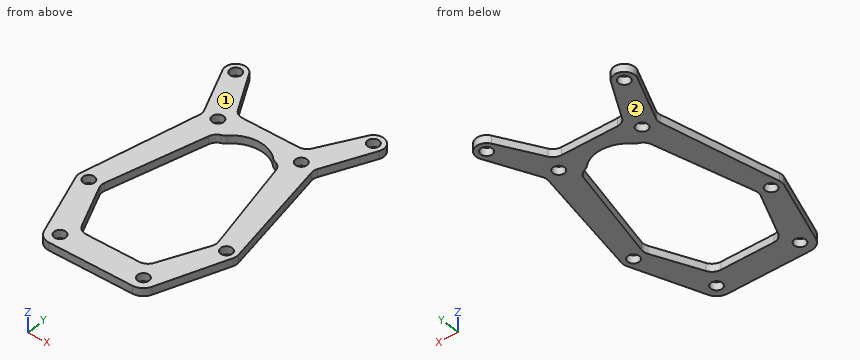
Autodesk Inventor part; units mm, degrees
ref_plane "YZ Plane" through (0, 0, 0) normal (1, 0, 0) x (0, 1, 0)
ref_plane "XZ Plane" through (0, 0, 0) normal (0, 1, 0) x (-1, 0, 0)
ref_plane "XY Plane" through (0, 0, 0) normal (0, 0, 1) x (1, 0, 0)
sketch "スケッチ1" plane through (0, 0, 0) normal (0, 0, 1) x (1, 0, 0)
  circle A0 centre (4, -6) radius 1.05
  circle A1 centre (4, -6) radius 1.1
  circle A2 centre (20, -6) radius 1.05
  circle A3 centre (20, -42) radius 1.1
  circle A4 centre (4, -42) radius 1.05
  circle A5 centre (20, -6) radius 1.1
  circle A6 centre (20, -42) radius 1.1
  circle A7 centre (4, -42) radius 1.1
  circle A8 centre (4, -42) radius 2.5
  circle A9 centre (20, -42) radius 2.5
  circle A10 centre (20, -6) radius 2.5
  circle A11 centre (4, -6) radius 2.5
  arc A12 (-0.741742, -29.885509) -> (-0.741742, -28.614491) centre (-1.2, -29.25) ccw
  arc A13 (24.741742, -28.614491) -> (24.741742, -29.885509) centre (25.2, -29.25) ccw
  arc A14 (-0.741742, 3.614491) -> (-0.741742, 4.885509) centre (-1.2, 4.25) ccw
  arc A15 (24.741742, 4.885509) -> (24.741742, 3.614491) centre (25.2, 4.25) ccw
  line L0 (24.741742, 5.75) -> (24.741742, 4.885509)
  line L1 (24.741742, 5.75) -> (22.7, 5.75)
  line L2 (22.7, 5.75) -> (22.7, 2.75)
  line L3 (24.741742, 2.75) -> (22.7, 2.75)
  line L4 (24.741742, 3.614491) -> (24.741742, 2.75)
  circle A16 centre (-1.2, 4.25) radius 1.1
  circle A17 centre (25.2, 4.25) radius 1.1
  circle A18 centre (25.2, -29.25) radius 1.1
  circle A19 centre (-1.2, -29.25) radius 1.1
  circle A20 centre (-1.2, -29.25) radius 2
  circle A21 centre (25.2, -29.25) radius 2
  circle A22 centre (25.2, 4.25) radius 2
  circle A23 centre (-1.2, 4.25) radius 2
  line L5 (-3.078107, -29.937542) -> (1.652366, -42.859427)
  line L6 (0.623256, -28.427966) -> (6.279069, -40.972458)
  line L7 (4, -39.5) -> (20, -39.5)
  line L8 (20, -44.5) -> (4, -44.5)
  line L9 (0.742189, -29.727393) -> (6.427736, -6.596741)
  line L10 (-3.160511, -28.854531) -> (1.549361, -5.505664)
  line L11 (-3.021278, 3.423595) -> (1.723402, -7.033006)
  line L12 (6.17819, -4.773016) -> (0.542552, 5.231587)
  line L13 (4, -3.5) -> (20, -3.5)
  line L14 (20, -8.5) -> (4, -8.5)
  line L15 (17.82181, -4.773016) -> (23.457448, 5.231587)
  line L16 (27.021278, 3.423595) -> (22.276598, -7.033006)
  line L17 (17.572264, -6.596741) -> (23.257811, -29.727393)
  line L18 (27.160511, -28.854531) -> (22.450639, -5.505664)
  line L19 (23.376744, -28.427966) -> (17.720931, -40.972458)
  line L20 (27.078107, -29.937542) -> (22.347634, -42.859427)
  circle A24 centre (12, -12.5) radius 6.232545
  point P0 (0, 0)
  point P1 (5.615196, -39.5)
  point P2 (0.906933, -29.057158)
  point P3 (5.959912, -8.5)
  point P4 (18.040088, -8.5)
  point P5 (23.093067, -29.057158)
  point P6 (18.384804, -39.5)
  point P7 (18.538906, -3.5)
  point P8 (5.461094, -3.5)
  point P9 (1.389644, -6.29745)
  point P10 (22.610356, -6.29745)
  point P11 (7.220396, -8.5)
  point P12 (16.779604, -8.5)
  dimension "d0" = 2.2
  dimension "d1" = 2.2
  dimension "d2" = 2.2
  dimension "d3" = 2.2
  dimension "d4" = 5
  dimension "d5" = 5
  dimension "d6" = 5
  dimension "d7" = 5
  dimension "d8" = 2.2
  dimension "d9" = 2.2
  dimension "d10" = 2.2
  dimension "d11" = 2.2
  dimension "d12" = 4
  dimension "d13" = 4
  dimension "d14" = 4
  dimension "d15" = 4
sketch "スケッチ1 outline for 押し出し1" plane through (0, 0, 0) normal (0, 0, 1) x (1, 0, 0)
  arc A0 (27.021278, 3.423595) -> (23.457448, 5.231587) centre (25.2, 4.25) ccw
  line L0 (22.610356, -6.29745) -> (27.021278, 3.423595)
  line L1 (23.457448, 5.231587) -> (18.538906, -3.5)
  line L2 (27.160511, -28.854531) -> (22.610356, -6.29745)
  line L3 (18.538906, -3.5) -> (5.461094, -3.5)
  arc A1 (27.078107, -29.937542) -> (27.160511, -28.854531) centre (25.2, -29.25) ccw
  line L4 (5.461094, -3.5) -> (0.542552, 5.231587)
  line L5 (22.347634, -42.859427) -> (27.078107, -29.937542)
  arc A2 (0.542552, 5.231587) -> (-3.021278, 3.423595) centre (-1.2, 4.25) ccw
  arc A3 (20, -44.5) -> (22.347634, -42.859427) centre (20, -42) ccw
  line L6 (-3.021278, 3.423595) -> (1.389644, -6.29745)
  line L7 (4, -44.5) -> (20, -44.5)
  line L8 (1.389644, -6.29745) -> (-3.160511, -28.854531)
  arc A4 (1.652366, -42.859427) -> (4, -44.5) centre (4, -42) ccw
  arc A5 (-3.160511, -28.854531) -> (-3.078107, -29.937542) centre (-1.2, -29.25) ccw
  line L9 (-3.078107, -29.937542) -> (1.652366, -42.859427)
  circle A6 centre (4, -42) radius 1.1
  circle A7 centre (-1.2, -29.25) radius 1.1
  circle A8 centre (20, -42) radius 1.1
  line L10 (5.615196, -39.5) -> (0.906933, -29.057158)
  line L11 (18.384804, -39.5) -> (5.615196, -39.5)
  line L12 (23.093067, -29.057158) -> (18.384804, -39.5)
  line L13 (18.040088, -8.5) -> (23.093067, -29.057158)
  line L14 (16.779604, -8.5) -> (18.040088, -8.5)
  arc A9 (7.220396, -8.5) -> (16.779604, -8.5) centre (12, -12.5) cw
  line L15 (5.959912, -8.5) -> (7.220396, -8.5)
  line L16 (0.906933, -29.057158) -> (5.959912, -8.5)
  circle A10 centre (25.2, -29.25) radius 1.1
  circle A11 centre (4, -6) radius 1.1
  circle A12 centre (-1.2, 4.25) radius 1.1
  circle A13 centre (20, -6) radius 1.1
  circle A14 centre (25.2, 4.25) radius 1.1
extrude "押し出し1" add sketch "スケッチ1 outline for 押し出し1" along normal blind 1.5
fillet "フィレット1" radius 2 12 edges at (0.9069, -29.0572, 0.75) (5.6152, -39.5, 0.75) (18.3848, -39.5, 0.75) (23.0931, -29.0572, 0.75) (18.0401, -8.5, 0.75) (5.9599, -8.5, 0.75) (7.2204, -8.5, 0.75) (16.7796, -8.5, 0.75) (5.4611, -3.5, 0.75) (18.5389, -3.5, 0.75) (1.3896, -6.2975, 0.75) (22.6104, -6.2975, 0.75)
properties part number "matasita" material "アルミニウム 2014-T4"
Could you check a few things on this model? Use its own coordinates, in mm. Face numbers are marked on the shaded views. Give positions to 0.01 mm unless a question says otherwise; leave off trailing zeros. Order: outer loops, then holes, each group sorted by start corner. A loop starts at its lowest first (then second) coordinate and runs counter-clockwise, first axis right, second up.
Q1. Suppose I cut it at C-C, the plane x = -1.2. Write out the boundary of the cut face in (y, z), and give its area (3 significant figures).
Q2. Suppose I cut it at B-B, the plane x = 11.5. Write out the boundary of the cut face in (y, z), and give its area (3 significant figures).
Q3. If I drill on line 1 along Y through (x, z) = (17, 0.65); line 2 along X through (y, z) = (-5, 1.3); line 3 along X through (y, z) = (-21.5, 0.5), over which ranges is the centre line in solid material (lowest first)?
Q4. I'm going to push a flat-ended pin straight in: P1, Ø2, axis at x = 20, y = -6, coming from the -Z side. Where does the tip first touch, or does it pass through?
Q5. Suppose I cut it at A-A, the plane y = -1. Write out the boundary of the cut face in (x, z), and give its area (3 significant figures).
Q6. Suppose I cut it at D-D, the plane y = 4.25. Write out the boundary of the cut face in (x, z), and give its area (3 significant figures).
Q7. We'd pull the mould along Z, two halves only. Please class the marked faces 1 and 2: +Z half, -Z half, draft (parallel to the pull), parting line (faces both ways), or undercut.
Solution:
1. outline: (-35.07, 0) - (-30.35, 0) - (-30.35, 1.5) - (-35.07, 1.5) - close; (-28.15, 0) - (-19.14, 0) - (-19.14, 1.5) - (-28.15, 1.5) - close; (-0.59, 0) - (3.15, 0) - (3.15, 1.5) - (-0.59, 1.5) - close; (5.35, 0) - (6.25, 0) - (6.25, 1.5) - (5.35, 1.5) - close
1. area: 27.6 mm2
2. outline: (-44.5, 0) - (-39.5, 0) - (-39.5, 1.5) - (-44.5, 1.5) - close; (-6.29, 0) - (-3.5, 0) - (-3.5, 1.5) - (-6.29, 1.5) - close
2. area: 11.7 mm2
3. line 1: y = -44.5 to -39.5, -8.4 to -3.5
3. line 2: x = 0.8 to 3.54, 4.46 to 19.54, 20.46 to 23.2
3. line 3: x = -1.68 to 2.76, 21.24 to 25.68
4. P1: passes through
5. outline: (-1.01, 0) - (4.05, 0) - (4.05, 1.5) - (-1.01, 1.5) - close; (19.95, 0) - (25.01, 0) - (25.01, 1.5) - (19.95, 1.5) - close
5. area: 15.2 mm2
6. outline: (-3.2, 0) - (-2.3, 0) - (-2.3, 1.5) - (-3.2, 1.5) - close; (-0.1, 0) - (1.1, 0) - (1.1, 1.5) - (-0.1, 1.5) - close; (22.9, 0) - (24.1, 0) - (24.1, 1.5) - (22.9, 1.5) - close; (26.3, 0) - (27.2, 0) - (27.2, 1.5) - (26.3, 1.5) - close
6. area: 6.29 mm2
7. face 1: +Z half
7. face 2: -Z half
